from build123d import *

# Parameters (mm, degrees)
F0_W      = 41
F0_H      = 20.1
F1_DEPTH  = 36.7
F3_DEPTH  = 2.5
F5_DEPTH  = 0.5
F6_R      = 6.55
F7_DEPTH  = 1
F8_R      = 5.375
F9_DEPTH  = 0.5
F12_DEPTH = 4.1
F13_SIZE  = 2
F15_W     = 6.85
F15_H     = 20.1
F16_DEPTH = 2.4
F18_DEPTH = 25
F19_R     = 0.1
F20_R     = 1.5
F21_DEPTH = 20
F23_DEPTH = 0.5


with BuildPart() as f1:
    # F0 (on Top) → F1 (new body)
    with BuildSketch(Plane.XY):
        with Locations((-10.45, 0)):
            Rectangle(F0_W, F0_H)
    extrude(amount=F1_DEPTH)

    # F2 (on face) → F3 (join)
    with BuildSketch(Plane.XY.offset(36.7)):
        with BuildLine():
            Line((-23.45, -10.05), (0, -10.05))
            ThreePointArc((0, -10.05), (10.05, 0), (0, 10.05))
            Line((0, 10.05), (-23.45, 10.05))
            Line((-23.45, 10.05), (-23.45, 4))
            ThreePointArc((-23.45, 4), (-25.45, 0), (-23.45, -4))
            Line((-23.45, -4), (-23.45, -10.05))
        make_face()
    extrude(amount=F3_DEPTH)

    # F4 (on face) → F5 (cut)
    with BuildSketch(Plane.XY.offset(39.2)):
        with BuildLine():
            Line((-23.45, -4), (-23.45, 4))
            ThreePointArc((-23.45, 4), (-25.45, 0), (-23.45, -4))
        make_face()
    extrude(amount=-F5_DEPTH, mode=Mode.SUBTRACT)

    # F6 (on face) → F7 (join)
    with BuildSketch(Plane.XY.offset(39.2)):
        Circle(F6_R)
    extrude(amount=F7_DEPTH)

    # F8 (on face) → F9 (join)
    with BuildSketch(Plane.XY.offset(40.2)):
        Circle(F8_R)
    extrude(amount=F9_DEPTH)

    # F11 (on face) → F12 (join)
    with BuildSketch(Plane.XY.offset(40.7)):
        Polygon((-0.2483938668, -2.8391548896), (0, -2.95), (0.2483938668, -2.8391548896), (0.5122621241, -2.9051828714), (0.7376342785, -2.7528886049), (1.0089594228, -2.7720932313), (1.204462046, -2.5829771931), (1.475, -2.5547749412), (1.6346928436, -2.3345833262), (1.8962234486, -2.2598311072), (2.0152543264, -2.0152543264), (2.2598311072, -1.8962234486), (2.3345833262, -1.6346928436), (2.5547749412, -1.475), (2.5829771931, -1.204462046), (2.7720932313, -1.0089594228), (2.7528886049, -0.7376342785), (2.9051828714, -0.5122621241), (2.8391548896, -0.2483938668), (2.95, 0), (2.8391548896, 0.2483938668), (2.9051828714, 0.5122621241), (2.7528886049, 0.7376342785), (2.7720932313, 1.0089594228), (2.5829771931, 1.204462046), (2.5547749412, 1.475), (2.3345833262, 1.6346928436), (2.2598311072, 1.8962234486), (2.0152543264, 2.0152543264), (1.8962234486, 2.2598311072), (1.6346928436, 2.3345833262), (1.475, 2.5547749412), (1.204462046, 2.5829771931), (1.0089594228, 2.7720932313), (0.7376342785, 2.7528886049), (0.5122621241, 2.9051828714), (0.2483938668, 2.8391548896), (0, 2.95), (-0.2483938668, 2.8391548896), (-0.5122621241, 2.9051828714), (-0.7376342785, 2.7528886049), (-1.0089594228, 2.7720932313), (-1.204462046, 2.5829771931), (-1.475, 2.5547749412), (-1.6346928436, 2.3345833262), (-1.8962234486, 2.2598311072), (-2.0152543264, 2.0152543264), (-2.2598311072, 1.8962234486), (-2.3345833262, 1.6346928436), (-2.5547749412, 1.475), (-2.5829771931, 1.204462046), (-2.7720932313, 1.0089594228), (-2.7528886049, 0.7376342785), (-2.9051828714, 0.5122621241), (-2.8391548896, 0.2483938668), (-2.95, 0), (-2.8391548896, -0.2483938668), (-2.9051828714, -0.5122621241), (-2.7528886049, -0.7376342785), (-2.7720932313, -1.0089594228), (-2.5829771931, -1.204462046), (-2.5547749412, -1.475), (-2.3345833262, -1.6346928436), (-2.2598311072, -1.8962234486), (-2.0152543264, -2.0152543264), (-1.8962234486, -2.2598311072), (-1.6346928436, -2.3345833262), (-1.475, -2.5547749412), (-1.204462046, -2.5829771931), (-1.0089594228, -2.7720932313), (-0.7376342785, -2.7528886049), (-0.5122621241, -2.9051828714), align=None)
    extrude(amount=F12_DEPTH)

    # F13
    f13_edges = [f1.edges().sort_by_distance(p)[0] for p in [
        (-10.45, 10.05, 0),
        (10.05, 0, 0),
        (-10.45, -10.05, 0),
        (-30.95, 0, 0),
    ]]
    chamfer(f13_edges, length=F13_SIZE)

    # F15 (on offset) → F16 (join)
    with BuildSketch(Plane.XY.offset(30.85)):
        Polygon((10.05, 10.05), (10.05, 0), (10.05, -10.05), (16.9, -10.05), (16.9, 10.05), align=None)
        with Locations((-34.375, 0)):
            Rectangle(F15_W, F15_H)
    extrude(amount=-F16_DEPTH)

    # F17 (on face) → F18 (cut)
    with BuildSketch(Plane.XY.offset(30.85)):
        with BuildLine():
            Line((-38.7193858624, 4.3), (-37.018211788, 4.3))
            ThreePointArc((-37.018211788, 4.3), (-32.75, 5.05), (-37.018211788, 5.8))
            Line((-37.018211788, 5.8), (-38.7193858624, 5.8))
            Line((-38.7193858624, 5.8), (-38.7193858624, 4.3))
        make_face()
        with BuildLine():
            Line((20.3046184033, 5.8), (16.118211788, 5.8))
            ThreePointArc((16.118211788, 5.8), (11.85, 5.05), (16.118211788, 4.3))
            Line((16.118211788, 4.3), (20.3046184033, 4.3))
            Line((20.3046184033, 4.3), (20.3046184033, 5.8))
        make_face()
        with BuildLine():
            Line((-38.7193858624, -4.3), (-38.7193858624, -5.8))
            Line((-38.7193858624, -5.8), (-37.018211788, -5.8))
            ThreePointArc((-37.018211788, -5.8), (-32.75, -5.05), (-37.018211788, -4.3))
            Line((-37.018211788, -4.3), (-38.7193858624, -4.3))
        make_face()
        with BuildLine():
            Line((16.118211788, -5.8), (20.3046184033, -5.8))
            Line((20.3046184033, -5.8), (20.3046184033, -4.3))
            Line((20.3046184033, -4.3), (16.118211788, -4.3))
            ThreePointArc((16.118211788, -4.3), (11.85, -5.05), (16.118211788, -5.8))
        make_face()
    extrude(amount=-F18_DEPTH, mode=Mode.SUBTRACT)

    # F19
    f19_edges = [f1.edges().sort_by_distance(p)[0] for p in [
        (-6.55, 0, 39.2),
        (-6.55, 0, 40.2),
        (-5.375, 0, 40.2),
        (-5.375, 0, 40.7),
    ]]
    fillet(f19_edges, radius=F19_R)

    # F20 (on face) → F21 (cut)
    with BuildSketch(Plane.XY.offset(44.8)):
        Circle(F20_R)
    extrude(amount=-F21_DEPTH, mode=Mode.SUBTRACT)

    # F22 (on face) → F23 (join)
    with BuildSketch(Plane.XY.offset(39.2)):
        with BuildLine():
            Line((-9.9580191225, 9.55), (-22.95, 9.55))
            Line((-22.95, 9.55), (-22.95, -9.55))
            Line((-22.95, -9.55), (-9.9580191225, -9.55))
            Line((-9.9580191225, -9.55), (-9.9580191225, -3.3863537817))
            ThreePointArc((-9.9580191225, -3.3863537817), (-9.15, 0), (-9.9580191225, 3.3863537817))
            Line((-9.9580191225, 3.3863537817), (-9.9580191225, 9.55))
        make_face()
    extrude(amount=F23_DEPTH)


solid = f1.part
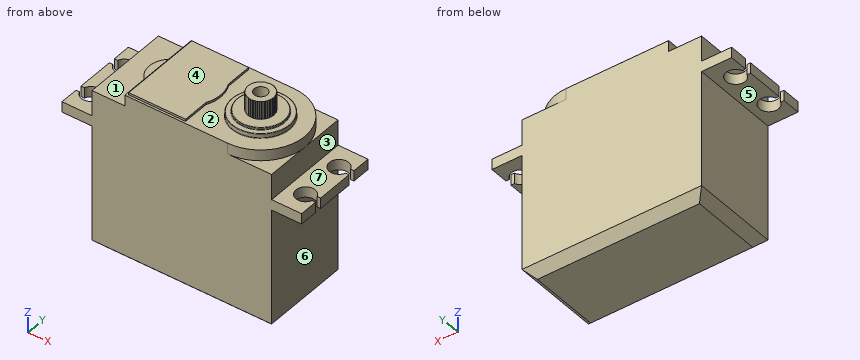
Design review of the part built by this model. Coordinates are the model's own, in mm. Face numbers are marked on the shaded views. A direction names the side the tool comes from. Give positions to 0.01 mm unless a question says otherwise; leave off trailing zeros. Order: outer loops, then holes, each group sorted by start corner. A loop starts at its lowest first (then second) coordinate and runs counter-clockwise, first axis right, second up.
1. For pin 1 Ø7.5 at (x, y) = (13.5, -4) entering from +Z; pin 2 Ø3 at (x, y) = (2.5, -6) entering from +Z; pin 3 Ø7 at (x, y) = (14.05, 5.05) entering from -Z, all flat-tipped, find the tip position at first contact; note any pin that passes through.
Solution:
pin 1: stops at z = 36.7
pin 2: stops at z = 40.7
pin 3: stops at z = 28.45
2. Tool access review of the marked faces 4, 5, 6 and 7: name each direction out of +Z, -Z, +X, -X, +Y, -Y from which nothing blocks a thin tool from reaching the whole face with its end or side.
Solution:
face 4: +Z, -X, +Y, -Y
face 5: -Z, -X, +Y, -Y
face 6: -Z, +X, +Y, -Y
face 7: +Z, +X, +Y, -Y
3. Mouldability with a two-part tool opening along X and no side actions: class the marked faces 1, 2 and 3 as +X half, -X half, draft (parallel to the pull), parting line (faces both ways), or undercut.
Solution:
face 1: draft
face 2: undercut
face 3: +X half
4. Add section C-C, the plane z = 18. State the section outline as (x, y) points.
Solution:
outline: (-30.95, -10.05) - (10.05, -10.05) - (10.05, 10.05) - (-30.95, 10.05) - close
5. Add section A-A, the plane x = -34.95. State the section outline as (y, z) points, then the cut area to 3 significant figures.
Solution:
outline: (-10.05, 28.45) - (-7.25, 28.45) - (-7.25, 30.85) - (-10.05, 30.85) - close; (-2.85, 28.45) - (2.85, 28.45) - (2.85, 30.85) - (-2.85, 30.85) - close; (7.25, 28.45) - (10.05, 28.45) - (10.05, 30.85) - (7.25, 30.85) - close
area: 27.1 mm2
6. Add section D-D, the plane x = 9. State the section outline as (y, z) points.
Solution:
outline: (-10.05, 2) - (-9, 0.95) - (9, 0.95) - (10.05, 2) - (10.05, 36.7) - (4.47, 36.7) - (4.47, 39.2) - (-4.47, 39.2) - (-4.47, 36.7) - (-10.05, 36.7) - close
7. To check wall thickness, follow L1, parallel to Y at x = 0, z = 33.5; L2, parallel to Y at x = -34, z = 29; L3, parallel to Z at x = -26, y = -1.25. State the ranges of each line that lie inside material, in increasing order.
Solution:
L1: y = -10.05 to -1.5, 1.5 to 10.05
L2: y = -10.05 to -7.03, -3.07 to 3.07, 7.03 to 10.05
L3: z = 0 to 36.7
8. Add section B-B, the plane x = -17.5. State the section outline as (y, z) points.
Solution:
outline: (-10.05, 2) - (-8.05, 0) - (8.05, 0) - (10.05, 2) - (10.05, 39.2) - (9.55, 39.2) - (9.55, 39.7) - (-9.55, 39.7) - (-9.55, 39.2) - (-10.05, 39.2) - close
